Can you work these out from the drawing? Everything is in mm from the part's minimum corner. Coordinates: 2 decimals unless noted, no trailing zeros. Write each loop counter-clockwise with the first axis right and the second up, starting at its lowest first coordinate (ties: lowest second). Pieces come first, ordered by that corner, then holes.
(1) For pin 1 Ø3 at (x, z) = (381, 2.5) entering from +Y; pin 2 Ø11 at (x, y) = (116.4, 130.5) entering from +Z; pin 3 Ø23.5 at (x, y) = (283.6, 130.5) entering from +Z; pin 4 Ø1.8 at (y, z) = (282.5, 3) entering from -X, each with a flat end and sliding along its axis, tell me the tip position at first contact or that it passes through.
(2) Please list where these lines run through material, in increasing order: probe 1 along Y at (x, z) = (116.4, 3.8); probe 2 along Y at (x, z) = (122, 3.5).
(3) Imagine slicing it at B-B, the plane y = 130.5. List the corners of the cut face in (x, z) for me, plus the area to 3 significant figures.
(4) Imagine slicing it at C-C, the plane z = 1. List the corners of the cut face in (x, y) for me.
(5) Imagine slicing it at A-A, the plane x = 309. List the corners of the cut face in (y, z) for me.
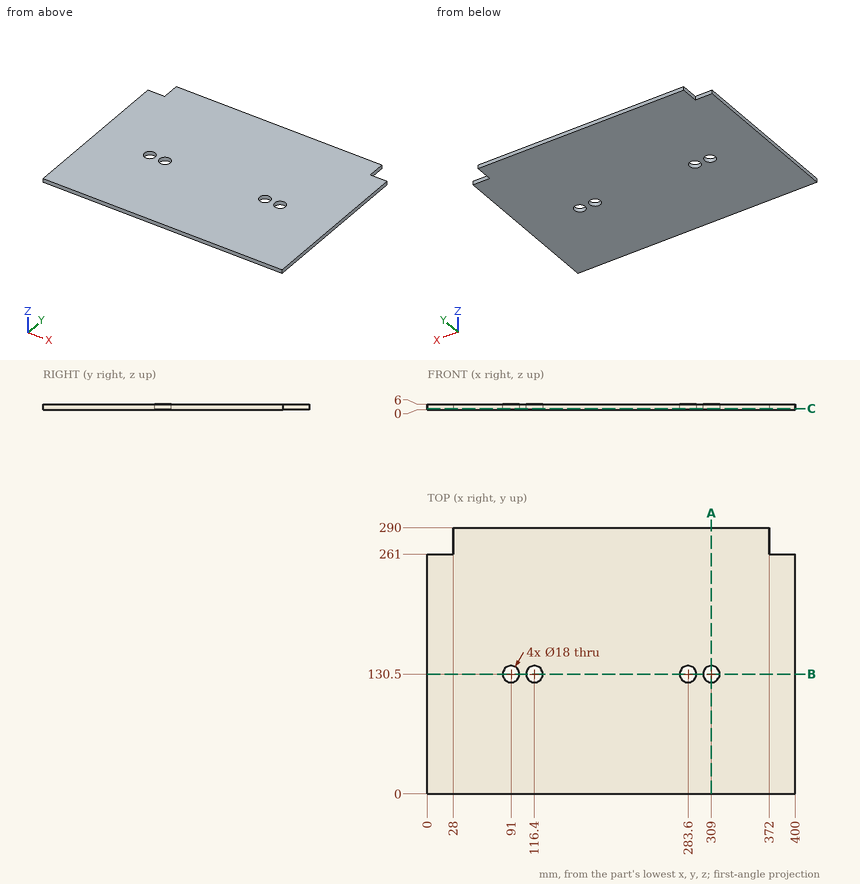
Recorded:
1. pin 1: stops at y = 261
1. pin 2: passes through
1. pin 3: stops at z = 6
1. pin 4: stops at x = 28
2. probe 1: y = 0 to 121.5, 139.5 to 290
2. probe 2: y = 0 to 123.45, 137.55 to 290
3. outline: (0, 0) - (82, 0) - (82, 6) - (0, 6) - close; (100, 0) - (107.4, 0) - (107.4, 6) - (100, 6) - close; (125.4, 0) - (274.6, 0) - (274.6, 6) - (125.4, 6) - close; (292.6, 0) - (300, 0) - (300, 6) - (292.6, 6) - close; (318, 0) - (400, 0) - (400, 6) - (318, 6) - close
3. area: 1,970 mm2
4. outline: (0, 0) - (400, 0) - (400, 261) - (372, 261) - (372, 290) - (28, 290) - (28, 261) - (0, 261) - close; hole circle Ø18 at (91, 130.5); hole circle Ø18 at (116.4, 130.5); hole circle Ø18 at (283.6, 130.5); hole circle Ø18 at (309, 130.5)
5. outline: (0, 0) - (121.5, 0) - (121.5, 6) - (0, 6) - close; (139.5, 0) - (290, 0) - (290, 6) - (139.5, 6) - close
